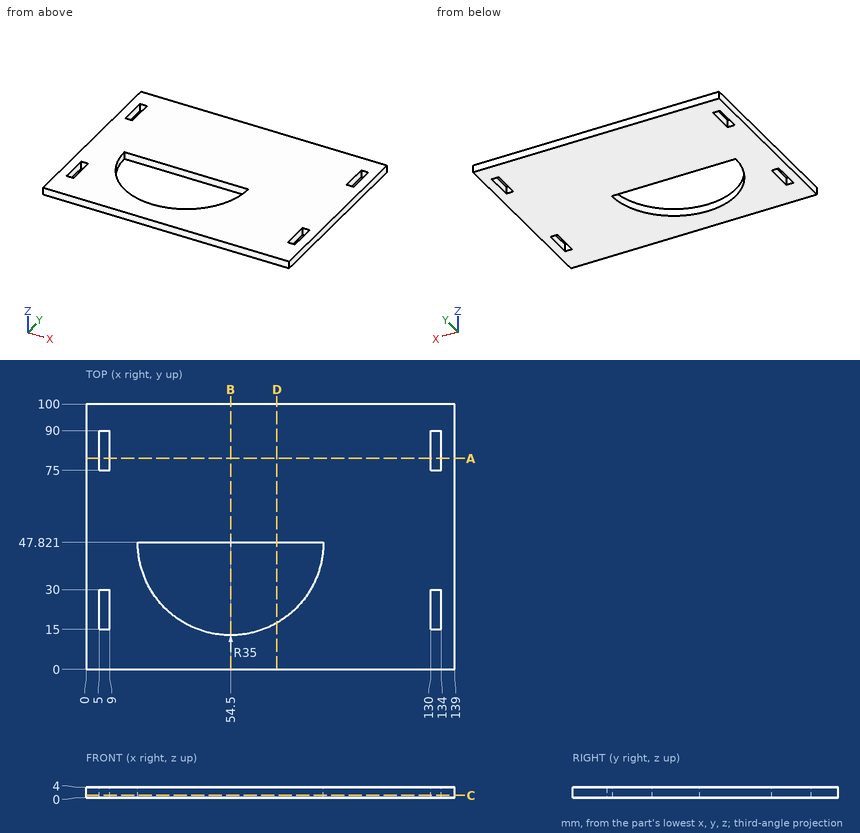
Job drawing, mm, ordinate dimensions from the low corner. One solid piece. Round coordinates to 2 decimals unless told otherwise and drop trailing zeros. Write each loop counter-clockwise with the first axis right and the second up, starting at its lowest first coordinate (ties: lowest second). Pieces come first, ordered by that corner, then holes. Notation, with made-up numbers: (70.5, 53.5) -> (109.5, 53.5) arc R14 ccw to (109.5, 77.5) -> close; hole circle Ø10 at (4, -20.5). An arc over 180 degrees is marked (long way). Answer as a JSON object with one key per item and string values.
(1) Probe probe 1 along X at (y, z) = (78.5, 1); probe 2 along Y at (x, z) = (30.5, 1.45) (1 decimal); probe 3 along Y at (x, z) = (77, 2.75). List the from-to ranges inside material, lowest first. Write a range as [from, to].
Reported:
{"probe 1": "x = [0, 5], [9, 130], [134, 139]", "probe 2": "y = [0, 22.3], [47.8, 100]", "probe 3": "y = [0, 21.01], [47.82, 100]"}
(2) Band-saw the part on C-C, the plane z = 0.9. List the corners of the cut face in (x, y).
Reported:
{"outline": "(0, 0) -> (139, 0) -> (139, 100) -> (0, 100) -> close; hole (5, 15) -> (9, 15) -> (9, 30) -> (5, 30) -> close; hole (5, 75) -> (9, 75) -> (9, 90) -> (5, 90) -> close; hole (19.5, 47.82) arc R35 ccw to (89.5, 47.82) -> close; hole (130, 15) -> (134, 15) -> (134, 30) -> (130, 30) -> close; hole (130, 75) -> (134, 75) -> (134, 90) -> (130, 90) -> close"}
(3) Band-saw the part on A-A, the plane y = 79.5. List the corners of the cut face in (x, z), then the cut area to 3 significant figures.
Reported:
{"outline": "(0, 0) -> (5, 0) -> (5, 4) -> (0, 4) -> close; (9, 0) -> (130, 0) -> (130, 4) -> (9, 4) -> close; (134, 0) -> (139, 0) -> (139, 4) -> (134, 4) -> close", "area": "524 mm^2"}
(4) Band-saw the part on B-B, the plane x = 54.5. List the corners of the cut face in (y, z), then the cut area to 3 significant figures.
Reported:
{"outline": "(0, 0) -> (12.82, 0) -> (12.82, 4) -> (0, 4) -> close; (47.82, 0) -> (100, 0) -> (100, 4) -> (47.82, 4) -> close", "area": "260 mm^2"}
(5) Pin check, flat tip, straight feed: P1, Ø1.5, axis at x = 25.5, z = 1, coming from the -Y side. Stop position of the tip, or through.
Reported:
{"P1": "stops at y = 0"}
(6) Band-saw the part on D-D, the plane x = 72. List the corners of the cut face in (y, z), then the cut area to 3 significant figures.
Reported:
{"outline": "(0, 0) -> (17.51, 0) -> (17.51, 4) -> (0, 4) -> close; (47.82, 0) -> (100, 0) -> (100, 4) -> (47.82, 4) -> close", "area": "279 mm^2"}
